The drawing under review shows one solid part. Ordinate dimensions are in mm from its lowest x, y, z. A direction names the side the tool comes from. Round coordinates to 2 decimals unless told otherwise and drop trailing zeros. Write each loop counter-clockwise with the first axis right and the second up, starting at its lowest first coordinate (ties: lowest second). Pieces come first, ordered by that corner, then holes. Notation, with made-up numbers: (-28, 3.25) -> (-14, 3.25) arc R12 cw to (-14, 21.25) -> close; hole circle Ø11 at (40, 45). An arc over 180 degrees is marked (long way). Use CSV: the item, a comma, the result in double quotes. Start each with the question number.
1) Machinability: for the marked faces 1, 2, 3 and 4, which of the approach directions +Z, -Z, +X, -X, +Y, -Y give a long, thin tool a straight path to every point of the face, cutting with its end or side? Answer none if there is none.
2) For pin 1 Ø1.5 at (x, y) = (4.5, 6) entering from -Z; pin 2 Ø1 at (x, z) = (2, 4) entering from -Y; pin 3 Ø1.6 at (x, z) = (3, 4.5) entering from +Y; pin 4 Ø2 at (y, z) = (7, 4) entering from +X, all flat-tipped, find the tip position at first contact; note any pin that passes through.
3) Take a section at B-B, the plane y = 11.75. Give the boundary of the cut face in (x, z), then the cut area to 3 significant figures.
4) Take a section at A-A, the plane x = 3.15. Give the boundary of the cut face in (y, z), then the cut area to 3 significant figures.
5) Take a section at C-C, the plane z = 3.75. Give the boundary of the cut face in (x, y).
6) Wall thickness on probe 1 along X at (y, z) = (5.75, 2.25); probe 2 along Z at (x, y) = (5.05, 11); probe 3 along Y at (x, z) = (3.4, 4): over which ranges is each line inside the solid? List them lowest first. Write a range as [from, to].
7) Take a section at D-D, the plane x = 4.75. Give the boundary of the cut face in (y, z).
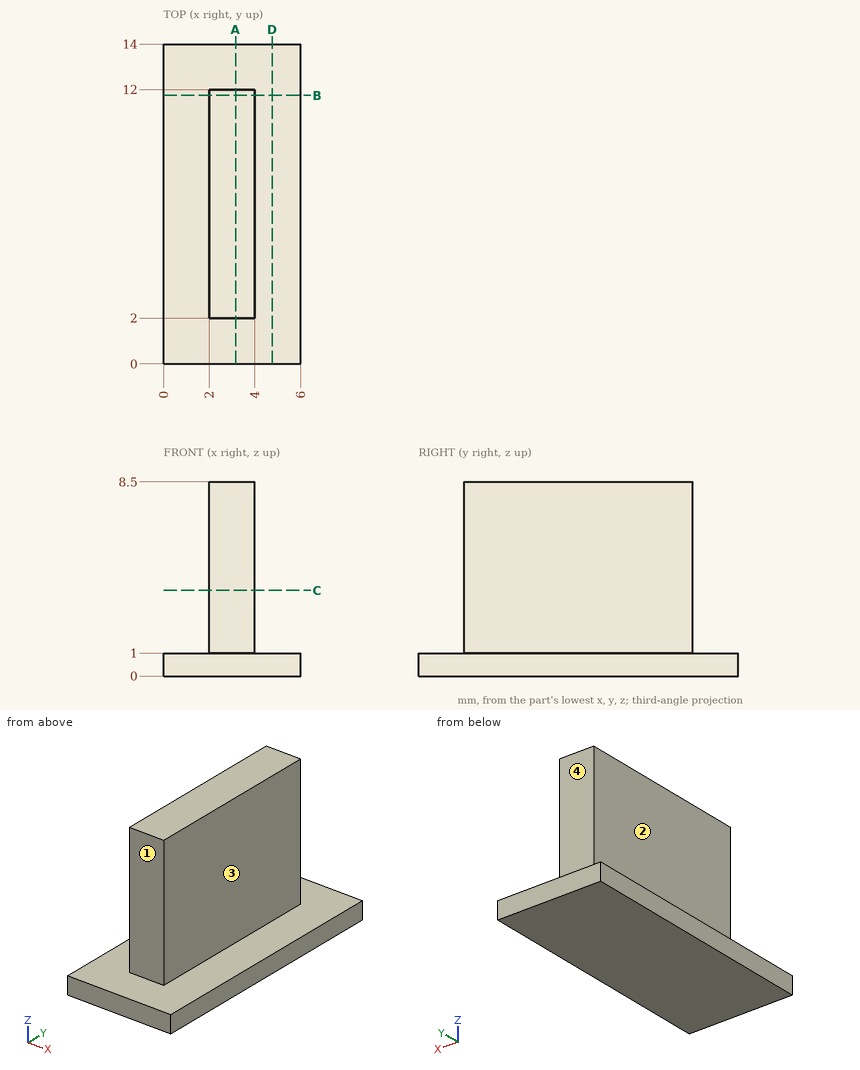
Values found:
1,face 1,"+Z, +X, -X, -Y"
1,face 2,"+Z, -X, +Y, -Y"
1,face 3,"+Z, +X, +Y, -Y"
1,face 4,"+Z, +X, -X, +Y"
2,pin 1,"z = 0"
2,pin 2,"y = 2"
2,pin 3,"y = 12"
2,pin 4,"x = 4"
3,outline,"(0, 0) -> (6, 0) -> (6, 1) -> (4, 1) -> (4, 8.5) -> (2, 8.5) -> (2, 1) -> (0, 1) -> close"
3,area,"21.0 mm²"
4,outline,"(0, 0) -> (14, 0) -> (14, 1) -> (12, 1) -> (12, 8.5) -> (2, 8.5) -> (2, 1) -> (0, 1) -> close"
4,area,"89.0 mm²"
5,outline,"(2, 2) -> (4, 2) -> (4, 12) -> (2, 12) -> close"
6,probe 1,"[2, 4]"
6,probe 2,"[0, 1]"
6,probe 3,"[2, 12]"
7,outline,"(0, 0) -> (14, 0) -> (14, 1) -> (0, 1) -> close"
